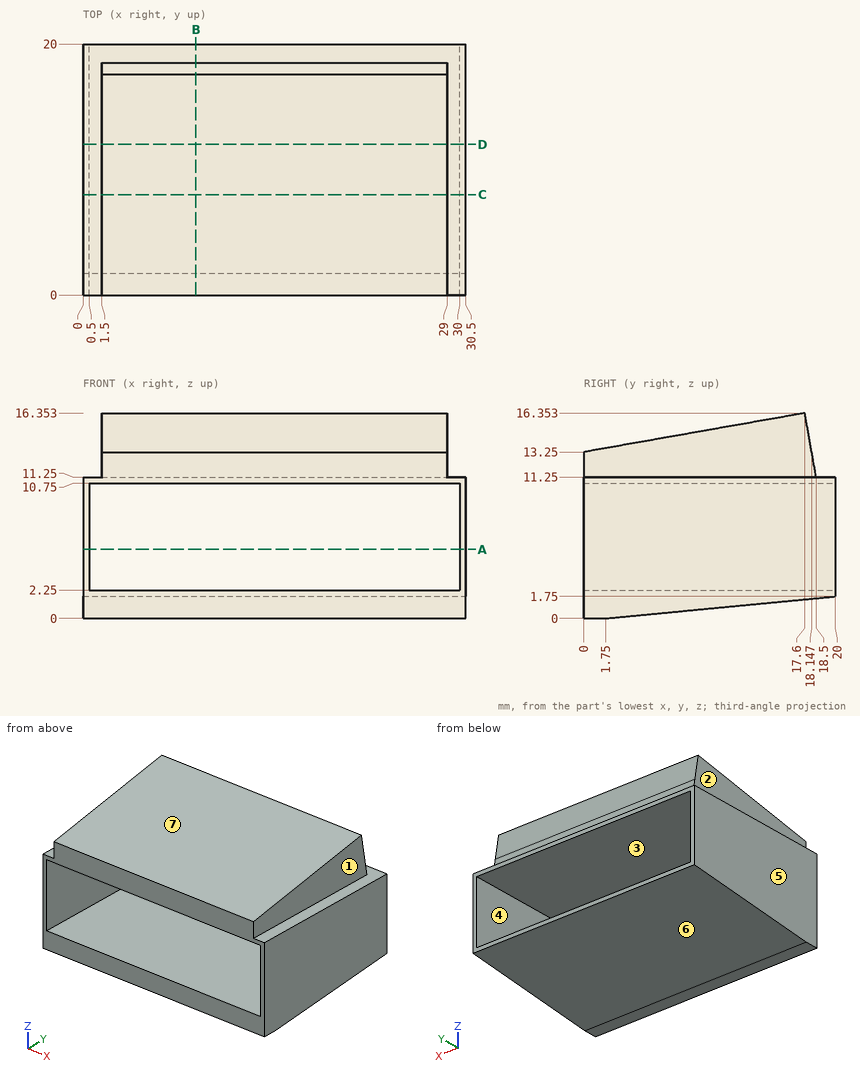
Verification items for this drawing (mm, ordinates from the low corner). A direction names the side the tool comes from. Coordinates: 2 decimals unless noted, no trailing zeros. Loops run counter-clockwise (first coordinate to the right, second up) from the corner with the lowest first, then second, coordinate; pieces in that order, holes last.
Item 1: Sectioned sample at D-D, the plane y = 12. Record the boundary of the cut face in (x, z).
Item 2: Go/stop test with flat-tipped pins: pin 1 Ø4 at (y, z) = (11.5, 13.5) entering from +X; pin 2 Ø2 at (x, z) = (4.5, 3.5) entering from +Y; pin 3 Ø4 at (y, z) = (9.5, 13) entering from -X; pin 4 Ø6 at (x, y) = (11.5, 9) entering from -Z. Record where each tip stops, or that it passes through.
Item 3: Sectioned sample at A-A, the plane z = 5.5. Record the boundary of the cut face in (x, y).
Item 4: Sectioned sample at C-C, the plane y = 8. Record the boundary of the cut face in (x, z), then the cut area to 3 significant figures.
Item 5: Release check for a two-part mould opening along Z. For the marked faces 4, 5, 6 and 7 record: released by +Z, released by -Z, zero draft, split by the parting line, or undercut.
Item 6: Thickness scan on line 1 (X direction, y = 12, z = 6.75); line 2 (X direction, y = 12.75, z = 13); line 3 (Z direction, x = 27, y = 4.25). Record the ranges inside material, lowest first.
Item 7: Access from +Z, -Z, +X, -X, +Y, -Y to the whole of each face (thin tool, end or side, straight path). Record for the marked faces 1, 2 and 3.
Item 8: Sectioned sample at B-B, the plane x = 9. Record the boundary of the cut face in (y, z), then the cut area to 3 significant figures.
Check result:
1. outline: (0, 0.98) - (30.5, 0.98) - (30.5, 11.25) - (29, 11.25) - (29, 15.37) - (1.5, 15.37) - (1.5, 11.25) - (0, 11.25) - close; hole (0.5, 2.25) - (30, 2.25) - (30, 10.75) - (0.5, 10.75) - close
2. pin 1: stops at x = 29
2. pin 2: passes through
2. pin 3: stops at x = 0
2. pin 4: stops at z = 0.41
3. outline: (0, 0) - (0.5, 0) - (0.5, 20) - (0, 20) - close; (30, 0) - (30.5, 0) - (30.5, 20) - (30, 20) - close
4. outline: (0, 0.6) - (30.5, 0.6) - (30.5, 11.25) - (29, 11.25) - (29, 14.66) - (1.5, 14.66) - (1.5, 11.25) - (0, 11.25) - close; hole (0.5, 2.25) - (30, 2.25) - (30, 10.75) - (0.5, 10.75) - close
4. area: 168 mm2
5. face 4: undercut
5. face 5: zero draft
5. face 6: released by -Z
5. face 7: released by +Z
6. line 1: x = 0 to 0.5, 30 to 30.5
6. line 2: x = 1.5 to 29
6. line 3: z = 0.24 to 2.25, 10.75 to 14
7. face 1: +Z, +X, +Y, -Y
7. face 2: +Z, -X, +Y, -Y
7. face 3: +Y, -Y
8. outline: (0, 0) - (1.75, 0) - (20, 1.75) - (20, 2.25) - (0, 2.25) - close; (0, 10.75) - (20, 10.75) - (20, 11.25) - (18.5, 11.25) - (17.6, 16.35) - (0, 13.25) - close
8. area: 104 mm2
